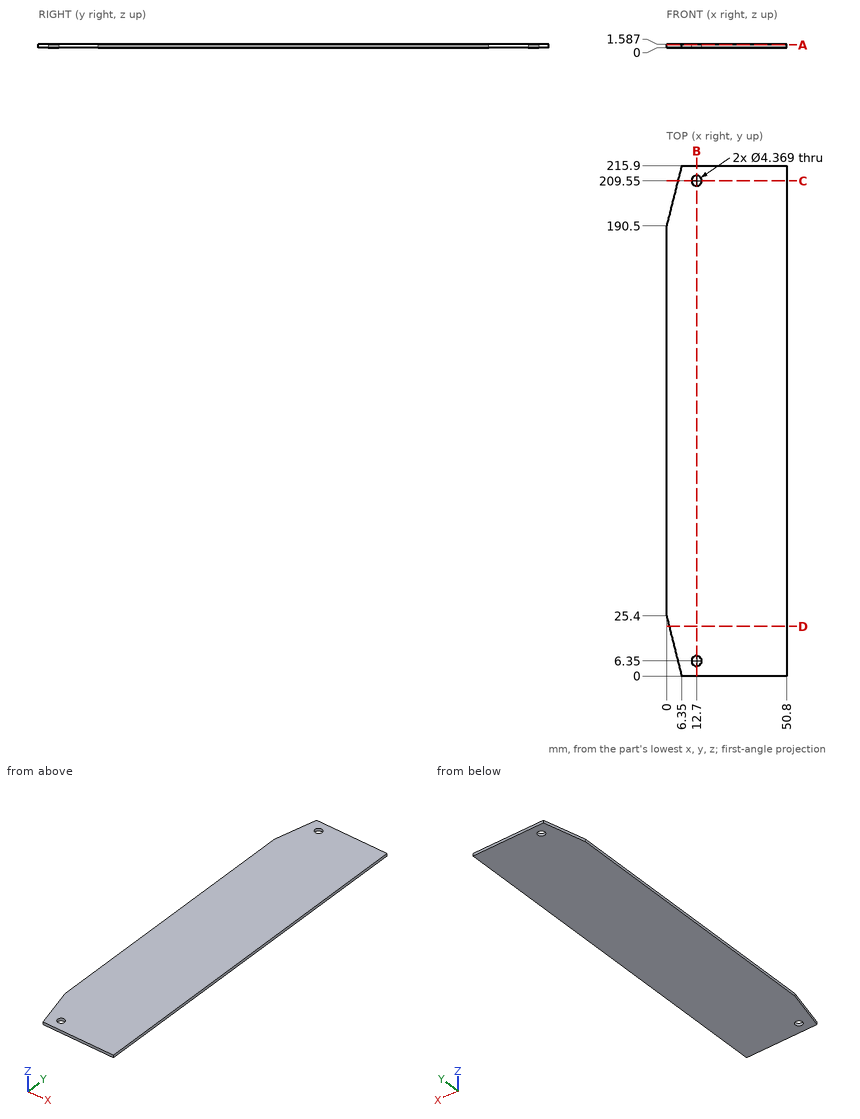
Source: three-view drawing plus pictorial views. Frame: mm from the lowest corner of the part. Give positions to 0.01 mm unless a question says otherwise; leave off trailing zeros. Order: outer loops, then holes, each group sorted by start corner. A loop starts at its lowest first (then second) coordinate and runs counter-clockwise, first axis right, second up. Notation, with made-up numbers: (88.5, 30) - (102.5, 30) arc R5 cw to (102.5, 36) - close; hole circle Ø1 at (65, -27.5). An arc over 180 degrees is marked (long way). Answer as a JSON object with one key per item and string values. Group by question number.
Q1. Cut plane D-D, the plane y = 21. Output: boundary loops of the cut face in (x, z).
Q2. Cut plane C-C, the plane y = 209.55. Output: boundary loops of the cut face in (x, z) (1 decimal).
Q3. Line query: probe 1 along Y at (x, z) = (12.7, 0.55) (1 decimal); probe 2 along X at (y, z) = (209.55, 0.85) (1 decimal); probe 3 along X at (y, z) = (15.5, 1.2) (1 decimal). Output: solid intervals per line, ascending.
Q4. Cut plane A-A, the plane z = 1.2. Count the separate pieces of the cut face and the enclosed holes in it, then the cut area to 3 significant figures.
Q5. Cut plane B-B, the plane x = 12.7. Output: boundary loops of the cut face in (y, z) (1 decimal).
Results:
{
 "1": {"outline": "(1.1, 0) - (50.8, 0) - (50.8, 1.59) - (1.1, 1.59) - close"},
 "2": {"outline": "(4.8, 0) - (10.5, 0) - (10.5, 1.6) - (4.8, 1.6) - close; (14.9, 0) - (50.8, 0) - (50.8, 1.6) - (14.9, 1.6) - close"},
 "3": {"probe 1": "0 to 4.2, 8.5 to 207.4, 211.7 to 215.9", "probe 2": "4.8 to 10.5, 14.9 to 50.8", "probe 3": "2.5 to 50.8"},
 "4": {"separate pieces": "1", "enclosed holes": "2", "area": "10,800 mm^2"},
 "5": {"outline": "(0, 0) - (4.2, 0) - (4.2, 1.6) - (0, 1.6) - close; (8.5, 0) - (207.4, 0) - (207.4, 1.6) - (8.5, 1.6) - close; (211.7, 0) - (215.9, 0) - (215.9, 1.6) - (211.7, 1.6) - close"}
}
